Model file for the job. Use its own axes, mm. Face numbers are marked on the shaded views. A direction names the side the tool comes from. Round coordinates to 2 decimals unless told otherwise and drop trailing zeros. Order: outer loops, then holes, each group sorted by start corner. A loop starts at its lowest first (then second) coordinate and runs counter-clockwise, first axis right, second up. Notation, with made-up numbers: (3, 87.5) - (20, 87.5) arc R11 ccw to (20, 105.5) - close; hole circle Ø5 at (86, 62.25). An arc over 180 degrees is marked (long way). Put each result on its own line as item: value. Start each with the question number.
Item 1: Saw through at D-D on y = -0.7. List the corners of the cut face in (x, z), plus the area to 3 significant figures.
Item 2: Mould opens along Z. For the marked faces 5, 6, 7 and 8 say: pulls with the +Z half, pulls with the -Z half, needs draft (parallel to the pull), parting line crosses it, or undercut.
Item 3: Saw through at C-C on y = -2.75. List the corners of the cut face in (x, z).
Item 4: Pin check, flat tips, straight feed: pin 1 Ø2.5 at (x, y) = (2.5, 0) entering from +Z; pin 2 Ø2 at (x, y) = (2, -3) entering from -Z; pin 3 Ø0.9 at (x, z) = (2, 3) entering from -Y. Stop position of each tip, or through.
Item 5: Probe probe 1 along Z at (x, y) = (1.5, -1); probe 2 along Z at (x, y) = (-2.5, -2.5); probe 3 along Z at (x, y) = (-3.75, 2.25). List the from-to ranges inside material, lowest first.
Item 6: Saw through at B-B on x = 2.5. List the corners of the cut face in (y, z), plus the area to 3 significant figures.
Item 7: Which spindle directions (+Z, -Z, +X, -X, +Y, -Y) get a long thin tool onto all of the face, cutting with end or side? Do the marked faces 1, 2, 3 and 4. Say none if no direction does.
Item 8: Saw through at A-A on z = 1.5. List the corners of the cut face in (x, y).
```python
from build123d import *
from build123d.topology import SkipClean

# Parameters (mm, degrees)
SKETCH_1_W             = 10
SKETCH_1_H             = 7.6
EXTRUDE_1_DEPTH        = 10
SKETCH_2_R             = 1.5
CUT_EXTRUDE_1_DEPTH    = 0.1
CUT_EXTRUDE_2_DEPTH    = 0.1
SKETCH_4_W             = 3
SKETCH_4_H             = 4.7
CUT_EXTRUDE_3_DEPTH    = 2
SKETCH_5_R             = 0.5
EXTRUDE_2_DEPTH        = 3
PATTERN_LINEAR_1_COUNT = 2
PATTERN_LINEAR_1_PITCH = 5
CHAMFER_1_SIZE         = 3.5
CHAMFER_1_SIZE2        = 1.632076804
CHAMFER_2_SIZE         = 2
CHAMFER_2_SIZE2        = 1.400415076


with BuildPart() as part:
    # Эскиз1 → Бобышка-Вытянуть1 (new body)
    with BuildSketch(Plane.XY):
        Rectangle(SKETCH_1_W, SKETCH_1_H)
    extrude(amount=EXTRUDE_1_DEPTH)

    # Эскиз2 → Вырез-Вытянуть1 (cut)
    with BuildSketch(Plane.XY.offset(10)):
        with Locations((2.5, 0)):
            Circle(SKETCH_2_R)
    cut_extrude_1 = extrude(amount=-CUT_EXTRUDE_1_DEPTH, mode=Mode.SUBTRACT)

    # Эскиз3 → Вырез-Вытянуть2 (cut)
    with SkipClean():  # the faces are left unmerged after this step: merging them gives an invalid solid
        with BuildSketch(Plane.XY.offset(9.9)):
            with BuildLine():
                Line((2.2, -1.469693846), (2.2, 1.469693846))
                ThreePointArc((2.2, 1.469693846), (2.5, 1.5), (2.8, 1.469693846))
                Line((2.8, 1.469693846), (2.8, -1.469693846))
                ThreePointArc((2.8, -1.469693846), (2.5, -1.5), (2.2, -1.469693846))
            make_face()
        cut_extrude_2 = extrude(amount=-CUT_EXTRUDE_2_DEPTH, mode=Mode.SUBTRACT)

    # Эскиз4 → Вырез-Вытянуть3 (cut)
    with SkipClean():  # the faces are left unmerged after this step: merging them gives an invalid solid
        with BuildSketch(Plane.XZ.offset(3.8)):
            with Locations((2.5, 2.85)):
                Rectangle(SKETCH_4_W, SKETCH_4_H)
        cut_extrude_3 = extrude(amount=-CUT_EXTRUDE_3_DEPTH, mode=Mode.SUBTRACT)

    # Эскиз5 → Бобышка-Вытянуть2 (add)
    with SkipClean():  # the faces are left unmerged after this step: merging them gives an invalid solid
        with BuildSketch(Plane(origin=(0, 0, 0), x_dir=(-1, 0, 0), z_dir=(0, 0, -1))):
            with Locations((-2.5, -0.7)):
                Circle(SKETCH_5_R)
        extrude_2 = extrude(amount=EXTRUDE_2_DEPTH)

    # Линейный массив1: Вырез-Вытянуть1, Вырез-Вытянуть2, Вырез-Вытянуть3, Бобышка-Вытянуть2 ×2
    with SkipClean():  # the faces are left unmerged after this step: merging them gives an invalid solid
        with Locations(*[(-i * PATTERN_LINEAR_1_PITCH, 0, 0) for i in range(1, PATTERN_LINEAR_1_COUNT)]):
            add(cut_extrude_1, mode=Mode.SUBTRACT)
            add(cut_extrude_2, mode=Mode.SUBTRACT)
            add(cut_extrude_3, mode=Mode.SUBTRACT)
            add(extrude_2)

    # Фаска1
    chamfer_1_edges = [part.edges().sort_by_distance(p)[0] for p in [
        (0, -3.8, 10),
    ]]
    chamfer_1_side = [part.faces().sort_by_distance(p)[0] for p in [
        (0, -3.8, 5.844428969),
    ]]
    chamfer(chamfer_1_edges, length=CHAMFER_1_SIZE, length2=CHAMFER_1_SIZE2, reference=chamfer_1_side[0])

    # Фаска2
    chamfer_2_edges = [part.edges().sort_by_distance(p)[0] for p in [
        (0, 3.8, 10),
    ]]
    chamfer_2_side = [part.faces().sort_by_distance(p)[0] for p in [
        (0, 3.8, 5),
    ]]
    chamfer(chamfer_2_edges, length=CHAMFER_2_SIZE, length2=CHAMFER_2_SIZE2, reference=chamfer_2_side[0])


solid = part.part
```
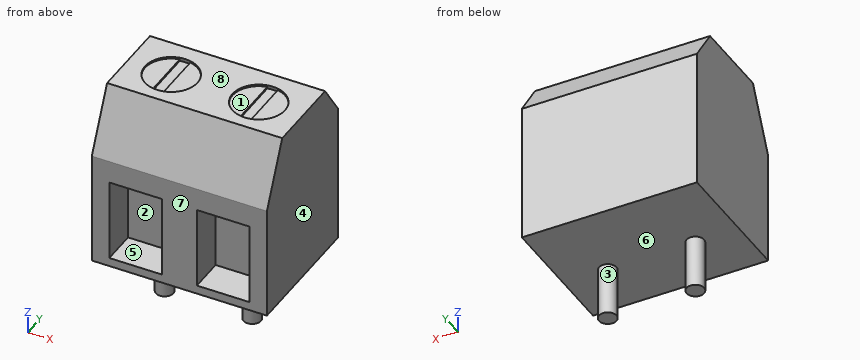
Results found:
1. outline: (-5, 0) - (-3, 0) - (-3, -3) - (-2, -3) - (-2, 0) - (2, 0) - (2, -3) - (3, -3) - (3, 0) - (5, 0) - (5, 10) - (3.83, 10) - (3.83, 9.9) - (2.8, 9.9) - (2.8, 9.8) - (2.2, 9.8) - (2.2, 9.9) - (1.17, 9.9) - (1.17, 10) - (-1.17, 10) - (-1.17, 9.9) - (-2.2, 9.9) - (-2.2, 9.8) - (-2.8, 9.8) - (-2.8, 9.9) - (-3.83, 9.9) - (-3.83, 10) - (-5, 10) - close
1. area: 105 mm²
2. face 5: undercut
2. face 6: pulls with the -Z half
2. face 7: needs draft
2. face 8: pulls with the +Z half
3. outline: (-5, 0) - (5, 0) - (5, 8.75) - (-5, 8.75) - close; hole (-4, 0.5) - (-1, 0.5) - (-1, 5.2) - (-4, 5.2) - close; hole (1, 0.5) - (4, 0.5) - (4, 5.2) - (1, 5.2) - close
4. pin 1: stops at z = 9.9
4. pin 2: stops at z = 0
4. pin 3: stops at y = -1.8
5. probe 1: z = 0 to 9.9
5. probe 2: z = 0 to 0.5, 5.2 to 9.29
5. probe 3: z = 0 to 10
6. outline: (-3.8, 0) - (-1.2, 0) - (-1.2, -3) - (-0.2, -3) - (-0.2, 0) - (3.8, 0) - (3.8, 8) - (2.4, 10) - (1.5, 10) - (1.5, 9.8) - (-1.5, 9.8) - (-1.5, 10) - (-2.17, 10) - (-3.8, 6.5) - (-3.8, 5.2) - (-1.8, 5.2) - (-1.8, 0.5) - (-3.8, 0.5) - close
6. area: 64.7 mm²
7. face 1: +Z
7. face 2: -Y
7. face 3: -Z
7. face 4: +Z, -Z, +X, +Y, -Y
8. outline: (-5, -3.8) - (-4, -3.8) - (-4, -1.8) - (-1, -1.8) - (-1, -3.8) - (1, -3.8) - (1, -1.8) - (4, -1.8) - (4, -3.8) - (5, -3.8) - (5, 3.8) - (-5, 3.8) - close
